from build123d import *

# Parameters (mm, degrees)
SKETCH1_R                            = 7.9375
BOSS_EXTRUDE1_DEPTH                  = 6.35
F_3_16_0_1875_DIAMETER_HOLE1_D       = 4.7625
SKETCH1_3_R                          = 7.9375
BOSS_EXTRUDE2_DEPTH                  = 9.525
W_0_386_DIAMETER_HOLE1_D             = 9.8044
FILLET1_R                            = 2
F_25_64_0_39063_DIAMETER_HOLE1_D     = 9.922002
F_25_64_0_39063_DIAMETER_HOLE1_DEPTH = 1.5875


with BuildPart() as part:
    # Sketch1 → Boss-Extrude1 (new body)
    with BuildSketch(Plane(origin=(0, 0, 0), x_dir=(1, 0, 0), z_dir=(0, 1, 0))):
        with BuildLine():
            ThreePointArc((2.26024053, 17.840513709), (0, 16.529128421), (-2.26024053, 17.840513709))
            Line((-2.26024053, 17.840513709), (-19.602540008, 56.648386542))
            ThreePointArc((-19.602540008, 56.648386542), (-27.954355314, 59.871226792), (-31.229481324, 51.539776269))
            Line((-31.229481324, 51.539776269), (-8.744221986, -0.519156562))
            ThreePointArc((-8.744221986, -0.519156562), (0, -6.267358068), (8.744221986, -0.519156562))
            Line((8.744221986, -0.519156562), (31.229481324, 51.539776269))
            ThreePointArc((31.229481324, 51.539776269), (27.954355314, 59.871226792), (19.602540008, 56.648386542))
            Line((19.602540008, 56.648386542), (2.26024053, 17.840513709))
        make_face()
        with Locations(Location((0, 3.257641932, 0), (0, 0, 270))):
            Circle(SKETCH1_R, mode=Mode.SUBTRACT)
    extrude(amount=BOSS_EXTRUDE1_DEPTH)

    # 3/16 (0.1875) Diameter Hole1 (through all)
    with Locations(Plane(origin=(0, 6.35, 0), x_dir=(1, 0, 0), z_dir=(0, 1, 0))):
        with Locations((-25.4, 54.057641932), (25.4, 54.057641932)):
            Hole(F_3_16_0_1875_DIAMETER_HOLE1_D / 2)

    # Sketch1<3> → Boss-Extrude2 (add)
    with BuildSketch(Plane(origin=(0, 0, 0), x_dir=(1, 0, 0), z_dir=(0, 1, 0))):
        with Locations(Location((0, 3.257641932, 0), (0, 0, 90))):
            Circle(SKETCH1_3_R)
    extrude(amount=BOSS_EXTRUDE2_DEPTH)

    # W (0.386) Diameter Hole1 (through all)
    with Locations(Plane(origin=(0, 9.525, 0), x_dir=(1, 0, 0), z_dir=(0, 1, 0))):
        with Locations((0, 3.257641932)):
            Hole(W_0_386_DIAMETER_HOLE1_D / 2)

    # Fillet1
    fillet1_edges = [part.edges().sort_by_distance(p)[0] for p in [
        (0, 6.35, 4.679858068),
    ]]
    fillet(fillet1_edges, radius=FILLET1_R)

    # 25/64 (0.39063) Diameter Hole1
    with Locations(Plane(origin=(0, 6.35, 0), x_dir=(1, 0, 0), z_dir=(0, 1, 0))):
        with Locations((-25.4, 54.057641932), (25.4, 54.057641932)):
            Hole(F_25_64_0_39063_DIAMETER_HOLE1_D / 2, depth=F_25_64_0_39063_DIAMETER_HOLE1_DEPTH)


solid = part.part
Geometry: final body of the model. Coordinates: model frame, mm. A direction names the side the tool comes from. Give positions to 0.01 mm unless a question says otherwise; leave off trailing zeros. Write each loop counter-clockwise with the first axis right and the second up, starting at its lowest first coordinate (ties: lowest second). Pieces come first, ordered by that corner, then holes. Notation, with made-up numbers: M -19,-7.75 L 32,-7.75 A17 ccw 32,20.25 Z; hole C 4,34.5 d7. An arc over 180 degrees is marked long. Answer in a Markdown table with one row per item. Add a question column.
(1) Reachability of faces 4 (the flat face through (19.83, 3.13, -25.15)), 5 (the flat face through (11.053, 3.131, -37.516)), 6 (the cylindrical face through (29.34, 5.55, -51.04)) from +Z, -Z, +X, -X, +Y, -Y: full face, straight path, thin tool, end or side. Return the list, or none.
(2) Ray query, line 1 (Z direction, x = 0, y = 4.5); line 2 (X direction, y = 5.5, z = -52.5); line 3 (Y direction, x = 6, z = -23). Return the intervals inside material, ascending.
(3) First-contact query: pin 1 (6 mm diameter, centred on x = 0, z = -3.26, fed in from -Y); pin 2 (1.5 mm diameter, centred on y = 3.5, z = -10.5, fed in from -X); pin 3 (3 mm diameter, centred on x = 28, z = -53, fed in from +Y); pin 4 (1 mm diameter, centred on y = 4, z = -2, fed in from -X). Flat tips, straight axial feed; report the tip coordinate or a pass-through.
(4) Section A-A on z = -20. Return loops of the section in (x, y).
(5) Section D-D on x = 21.5. Return loops of the section in (y, z).
(6) Mould query, pull axis X, two halves, no side actions, for faces 1 (the cylindrical face through (7.75, 8.91, -1.54)), 2 (the flat face through (27, 4.762, -52)), 3 (the flat face through (-10, 6.35, -31)). Classes: +X half, -X half, draft (parallel to the pull), parting line (faces both ways), or undercut.
(7) Section B-B on x = -25.4. Return loops of the section in (y, z).
(8) Section C-C on y = 2.75. State how many separate pieces and enclosed holes the cut face has, and give its area (3 significant figures).
Result set:
| question | item | result |
|---|---|---|
| 1 | face 4 | +Z, +X, +Y, -Y |
| 1 | face 5 | -Z, +Y, -Y |
| 1 | face 6 | +Y |
| 2 | line 1 | z = -16.53 to -8.16, 1.64 to 6.27 |
| 2 | line 2 | x = -31.56 to -30.11, -20.69 to -17.75, 17.75 to 20.69, 30.11 to 31.56 |
| 2 | line 3 | y = 0 to 6.35 |
| 3 | pin 1 | passes through |
| 3 | pin 2 | stops at x = -13.83 |
| 3 | pin 3 | stops at y = 4.76 |
| 3 | pin 4 | stops at x = -10.05 |
| 4 | outline | M -17.61,0 L -3.23,0 L -3.23,6.35 L -17.61,6.35 Z; M 3.23,0 L 17.61,0 L 17.61,6.35 L 3.23,6.35 Z |
| 5 | outline | M 0,-59.07 L 6.35,-59.07 L 6.35,-57.12 L 4.76,-57.12 L 4.76,-50.99 L 6.35,-50.99 L 6.35,-29.01 L 0,-29.01 Z |
| 6 | face 1 | parting line |
| 6 | face 2 | undercut |
| 6 | face 3 | draft |
| 7 | outline | M 0,-60.41 L 6.35,-60.41 L 6.35,-59.02 L 4.76,-59.02 L 4.76,-56.44 L 0,-56.44 Z; M 0,-51.68 L 4.76,-51.68 L 4.76,-49.1 L 6.35,-49.1 L 6.35,-38.04 L 0,-38.04 Z |
| 8 | separate pieces | 1 |
| 8 | enclosed holes | 3 |
| 8 | area | 1,580 mm^2 |
